```python
from build123d import *

# Parameters (mm, degrees)
SKETCH1_W                = 10
SKETCH1_H                = 70
REVOLVE1_ANGLE           = 40
CUT_EXTRUDE1_DEPTH       = 72.002236522
BOSS_EXTRUDE1_REACH      = 73.45
BOSS_EXTRUDE1_END_RADIUS = 8
SKETCH4_R                = 2.1


with BuildPart() as part:
    # Sketch1 → Revolve1 (revolve)
    with BuildSketch(Plane(origin=(0, 0, 0), x_dir=(0, 0, -1), z_dir=(1, 0, 0))):
        with Locations((5, 35)):
            Rectangle(SKETCH1_W, SKETCH1_H)
    revolve(axis=Axis((0, 0, 0), (0, 1, 0)), revolution_arc=REVOLVE1_ANGLE)

    # Sketch2 → Cut-Extrude1 (cut, through all)
    with BuildSketch(Plane(origin=(0, 70, 0), x_dir=(1, 0, 0), z_dir=(0, 1, 0))):
        with BuildLine():
            Line((-5.142300877, 6.128355545), (0, 0))
            Line((0, 0), (0, 8))
            ThreePointArc((0, 8), (-2.736161147, 7.517540966), (-5.142300877, 6.128355545))
        make_face()
    extrude(amount=-CUT_EXTRUDE1_DEPTH, mode=Mode.SUBTRACT)

    # Boss-Extrude1: up to this cylinder (the profile starts inside it)
    boss_extrude1_end = Plane(origin=(0, 35, 0), z_dir=(0, 1, 0)) * Cylinder(BOSS_EXTRUDE1_END_RADIUS, 203.9, mode=Mode.PRIVATE)
    # Sketch4 → Boss-Extrude1 (add, up to the surface)
    with BuildSketch(Plane(origin=(0.849050995, 0, 2.332748435), x_dir=(0.9396926207859081, 0, -0.34202014332566977), z_dir=(0.34202014332566977, 0, 0.9396926207859081)), mode=Mode.PRIVATE) as boss_extrude1_sk1:
        with Locations((0, 55)):
            Circle(SKETCH4_R)
    boss_extrude1_tool1 = extrude(boss_extrude1_sk1.sketch, amount=-BOSS_EXTRUDE1_REACH, mode=Mode.PRIVATE) & boss_extrude1_end
    add(boss_extrude1_tool1.solids().sort_by_distance((0.849051, 55, 2.332748))[0])
    # Sketch4 → Boss-Extrude1 (add, up to the surface)
    with BuildSketch(Plane(origin=(0.849050995, 0, 2.332748435), x_dir=(0.9396926207859081, 0, -0.34202014332566977), z_dir=(0.34202014332566977, 0, 0.9396926207859081)), mode=Mode.PRIVATE) as boss_extrude1_sk2:
        with Locations((0, 15)):
            Circle(SKETCH4_R)
    boss_extrude1_tool2 = extrude(boss_extrude1_sk2.sketch, amount=-BOSS_EXTRUDE1_REACH, mode=Mode.PRIVATE) & boss_extrude1_end
    add(boss_extrude1_tool2.solids().sort_by_distance((0.849051, 15, 2.332748))[0])


solid = part.part
```
Design review of the part built by this model. Coordinates are the model's own, in mm. Coordinates: 2 decimals unless noted, no trailing zeros. Loops run counter-clockwise (first coordinate to the right, second up) from the corner with the lowest first, then second, coordinate; pieces in that order, holes last.
Q1. To check wall thickness, follow line 1 (Y direction, x = 2, z = 0); line 2 (Y direction, x = -0.5, z = -1.5); line 3 (Z direction, x = -2.75, y = 12). State the ranges of each line that lie inside material, in increasing order.
Reported:
line 1: y = 14.06 to 15.94, 54.06 to 55.94
line 2: y = 12.9 to 17.1, 52.9 to 57.1
line 3: z = -9.61 to -7.51
Q2. The part is to be moulded in two halves that separate along Y. For faces 1 (the face through (-2.7, 35.49, -7.53)), 2 (the face through (-5.776, 35.49, -6.884)), 3 (the face through (-3, 70, -9)), say which applies: +Y half, -Y half, draft (parallel to the pull), parting line (faces both ways), or undercut.
Reported:
face 1: undercut
face 2: draft
face 3: +Y half
Q3. We need section B-B on z = -8.75. State the section outline as (x, y) points, and give its area (3 significant figures).
Reported:
outline: (-4.84, 0) - (0, 0) - (0, 70) - (-4.84, 70) - close
area: 339 mm2
Q4. For pin 1 (2 mm diameter, centred on y = 54, z = -3.5, fed in from +X); pin 2 (3 mm diameter, centred on x = -1.5, z = -2.5, fed in from +Y); pin 3 (0.6 mm diameter, centred on y = 19.5, z = -9.5, fed in from +X), all flat-tipped, find the tip position at first contact; note any pin that passes through.
Reported:
pin 1: stops at x = 1.21
pin 2: stops at y = 57.1
pin 3: stops at x = 0
Q5. We need section A-A on y = 56. State the section outline as (x, z) points, and give its area (3 significant figures).
Reported:
outline: (-6.43, -7.66) arc R10 ccw to (0, -10) - (0, -8) arc R8 cw to (-0.93, -7.95) - (2.58, 1.7) - (-0.89, 2.96) - (-4.4, -6.68) arc R8 cw to (-5.14, -6.13) - close
area: 51.0 mm2
